The model under review builds one solid part; all positions refer to its coordinate system, in mm. A direction names the side the tool comes from. Round coordinates to 2 decimals unless told otherwise and drop trailing zeros. Write each question's results on one line, items separated by ' | '. Start each with the question number.
Item 1: Tool access review of faces 5 (the flat face through (4, 16, -841.375)), 6 (the flat face through (-4, 12.7, 232)): name each direction out of +Z, -Z, +X, -X, +Y, -Y from which nothing blocks a thin tool from reaching the whole face with its end or side.
Item 2: For L1, parallel to X at y = 11.5, z = 6.5; L2, parallel to Y at x = -23.5, z = -219.5 (3 decimals), list the stretches that pass through material, from the lowest coordinate up. Write a range as from..to.
Item 3: Mouldability with a two-part tool opening along X and no side actions: class faces 1 (the flat face through (-4, 12.7, 460)), 2 (the flat face through (-4, 12.7, 155)), 3 (the flat face through (273.05, 16, -9)), 4 (the flat face through (-4, 31.75, -9)) as pulls with the +X half, pulls with the -X half, needs draft (parallel to the pull), parting line crosses it, or undercut.
Item 4: Clearance check with flat-ended pins moving along their axes: pin 1 Ø10 at (x, z) = (-94, 3) entering from -Y (3 decimals); pin 2 Ø16.5 at (x, z) = (87.5, 386) entering from -Y. State where each tip first meets the part, or that it passes through.
from build123d import *

# Parameters (mm, degrees)
F0_W      = 533.4
F0_H      = 1682.75
F1_DEPTH  = 31.75
F3_DEPTH  = 635
F21_W     = 31.75
F21_H     = 1682.75
F22_DEPTH = 6.35
F23_W     = 31.75
F23_H     = 1682.75
F24_DEPTH = 6.35
F25_W     = 546.1
F25_H     = 31.75
F26_DEPTH = 6.35
F27_R     = 1.5875


with BuildPart() as f1:
    # F0 (on Front) → F1 (new body)
    with BuildSketch(Plane.XZ):
        Rectangle(F0_W, F0_H)
    extrude(amount=-F1_DEPTH)


with BuildPart() as f3:
    # F2 (on face) → F3 (new body)
    with BuildSketch(Plane.YZ.offset(266.7)):
        Polygon((-6.35, -6.35), (-4.7625, -4.7625), (-3.175, -4.7625), (0, -6.5955926), (0, -14.9672802), (6.35, -16.66875), (6.35, 16.66875), (0, 14.9672548), (0, 6.5955672), (-3.175, 4.7625), (-4.7625, 4.7625), (-6.35, 6.35), align=None)
    extrude(amount=F3_DEPTH)


with BuildPart() as f6_1:
    # F6: copy of F3
    add(f3.part.moved(Location((-635, 6.35, -225.425))))


with BuildPart() as f7_1:
    # F7: copy of F3
    add(f3.part.moved(Location((-635, 6.35, -149.225))))


with BuildPart() as f8_1:
    # F8: copy of F3
    add(f3.part.moved(Location((-635, 6.35, -73.025))))


with BuildPart() as f9_1:
    # F9: copy of F3
    add(f3.part.moved(Location((-635, 6.35, 3.175))))


with BuildPart() as f10_1:
    # F10: copy of F3
    add(f3.part.moved(Location((-635, 6.35, 79.375))))


with BuildPart() as f11_1:
    # F11: copy of F3
    add(f3.part.moved(Location((-635, 6.35, 155.575))))


with BuildPart() as f12_1:
    # F12: copy of F3
    add(f3.part.moved(Location((-635, 6.35, 231.775))))


with BuildPart() as f13_1:
    # F13: copy of F3
    add(f3.part.moved(Location((-635, 6.35, 307.975))))


with BuildPart() as f14_1:
    # F14: copy of F3
    add(f3.part.moved(Location((-635, 6.35, 384.175))))


with BuildPart() as f15_1:
    # F15: copy of F3
    add(f3.part.moved(Location((-635, 6.35, 460.375))))


with BuildPart() as f16_1:
    # F16: copy of F3
    add(f3.part.moved(Location((-635, 6.35, 536.575))))


with BuildPart() as f17_1:
    # F17: copy of F3
    add(f3.part.moved(Location((-635, 6.35, 612.775))))


with BuildPart() as f18_1:
    # F18: copy of F3
    add(f3.part.moved(Location((-635, 6.35, 688.975))))


with BuildPart() as f3_1:
    # F19: moved
    add(f3.part.moved(Location((-635, 6.35, 765.175))))


with BuildPart() as f1_1:
    add(f1.part)

    # F20: cut F3, F18_1, F17_1, F16_1, F15_1, F14_1, F13_1, F12_1, F11_1, F10_1, F9_1, F8_1, F7_1, F6_1
    add(f3_1.part, mode=Mode.SUBTRACT)
    add(f18_1.part, mode=Mode.SUBTRACT)
    add(f17_1.part, mode=Mode.SUBTRACT)
    add(f16_1.part, mode=Mode.SUBTRACT)
    add(f15_1.part, mode=Mode.SUBTRACT)
    add(f14_1.part, mode=Mode.SUBTRACT)
    add(f13_1.part, mode=Mode.SUBTRACT)
    add(f12_1.part, mode=Mode.SUBTRACT)
    add(f11_1.part, mode=Mode.SUBTRACT)
    add(f10_1.part, mode=Mode.SUBTRACT)
    add(f9_1.part, mode=Mode.SUBTRACT)
    add(f8_1.part, mode=Mode.SUBTRACT)
    add(f7_1.part, mode=Mode.SUBTRACT)
    add(f6_1.part, mode=Mode.SUBTRACT)

    # F21 (on face) → F22 (join)
    with BuildSketch(Plane.YZ.offset(266.7)):
        with Locations((15.875, 0)):
            Rectangle(F21_W, F21_H)
    extrude(amount=F22_DEPTH)

    # F23 (on face) → F24 (join)
    with BuildSketch(Plane(origin=(-266.7, 0, 0), x_dir=(0, -1, 0), z_dir=(-1, 0, 0))):
        with Locations((-15.875, 0)):
            Rectangle(F23_W, F23_H)
    extrude(amount=F24_DEPTH)

    # F25 (on face) → F26 (join)
    with BuildSketch(Plane.XY.offset(841.375)):
        with Locations((0, 15.875)):
            Rectangle(F25_W, F25_H)
    extrude(amount=F26_DEPTH)

    # F27
    f27_edges = [f1_1.edges().sort_by_distance(p)[0] for p in [
        (0, 31.75, 847.725),
        (0, 0, 847.725),
        (-273.05, 31.75, 3.175),
        (-273.05, 0, 3.175),
        (273.05, 0, 3.175),
        (273.05, 31.75, 3.175),
        (273.05, 15.875, 847.725),
        (-273.05, 15.875, 847.725),
    ]]
    fillet(f27_edges, radius=F27_R)


solid = f1_1.part
Here are the results:
1) face 5: -Z, +X, -X, +Y, -Y | face 6: none
2) L1: x = -273.05..-266.7, 266.7..273.05 | L2: y = 0.425..5.189, 12.7..31.75
3) face 1: undercut | face 2: undercut | face 3: pulls with the +X half | face 4: needs draft
4) pin 1: stops at y = 1.175 | pin 2: stops at y = 0
